The listing builds one solid part. Answer for the finished solid, in the listing's coordinates (mm). Face numbers are marked on the shaded views. Round coordinates to 2 decimals unless told otherwise and drop trailing zeros. Write each loop counter-clockwise with the first axis right and the second up, starting at its lowest first coordinate (ties: lowest second). Pieces come first, ordered by that corner, then holes.
(1) A cutting plane is placed at A-A, the plane z = 16.5. Give the vertices of the cut face in (x, y).
(2) Find the intervals of material crossed by probe 1 along Y at (x, z) = (1.5, 15.5); probe 2 along Y at (x, z) = (1.5, 18); probe 3 along X at (y, z) = (-1.25, 34.5), in increasing order.
(3) The mould has two halves that part along Y. Classify the marked faces 1 and 2: +Y half, -Y half, draft (parallel to the pull), parting line (faces both ways), or undercut.
(4) Each of these flat-tipped pins is pushed along its axis until it touches: pin 1 Ø4.5 at (x, y) = (-1.5, 1) entering from +Z; pin 2 Ø2 at (x, z) = (-1.5, 23) entering from -Y. Where does it stop, or does it pass through?
(5) A cutting plane is placed at B-B, the plane z = 24. Give the vertices of the cut face in (x, y), and give its area (3 significant figures).
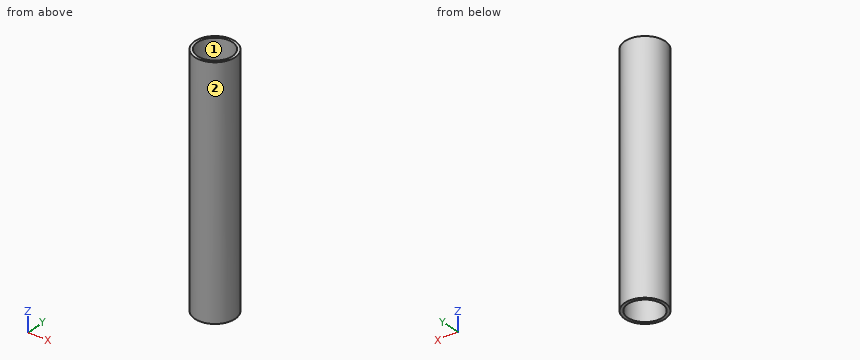
from build123d import *

# Parameters (mm, degrees)
F0_R     = 3.75
F1_DEPTH = 45
F2_R     = 3.25
F3_DEPTH = 22.5
F5_R     = 3.25
F6_DEPTH = 22.5
F7_SIZE2 = 0.49999
F7_SIZE  = 22.49999


# Not quite as in the source:
# - a fillet or chamfer that OpenCascade refuses, or shapes differently, is made with other operations: its cross-section is extruded or revolved along the edge and cut away or added
# - a fillet or chamfer is up to 0.001 mm smaller than in the source, because OpenCascade refuses the exact size


with BuildPart() as f1:
    # F0 (on Top) → F1 (new body)
    with BuildSketch(Plane.XY):
        Circle(F0_R)
    extrude(amount=F1_DEPTH)

    # F2 (on face) → F3 (cut)
    with BuildSketch(Plane.XY):
        Circle(F2_R)
    extrude(amount=F3_DEPTH, mode=Mode.SUBTRACT)

    # F4: chamfer of 25 x 0.5 on 1 edges, made by hand


with BuildPart() as f4_tool2:
    # F4_s3 → F4_t4 (revolve)
    with BuildSketch(Plane.XZ):
        Polygon((3.25, -2.5), (2.75, 22.5), (3.25, 22.5), align=None)
    revolve(axis=Axis((0, 0, 22.5), (0, 0, 1)))

    split(bisect_by=Plane.XY, keep=Keep.TOP)


with BuildPart() as f1_1:
    add(f1.part)

    # F4_t1: union F4_tool2
    add(f4_tool2.part)

    # F5 (on face) → F6 (cut)
    with BuildSketch(Plane.XY.offset(45)):
        Circle(F5_R)
    extrude(amount=-F6_DEPTH, mode=Mode.SUBTRACT)

    # F7 (size 22.5 and 0.5 in the source; OpenCascade refuses exactly that, so slightly less here)
    f7_edges = [f1_1.edges().sort_by_distance(p)[0] for p in [
        (-3.25, 0, 22.5),
    ]]
    f7_side = f1_1.faces().sort_by_distance((-3.25, 0, 33.75))[0]
    chamfer(f7_edges, length=F7_SIZE, length2=F7_SIZE2, reference=f7_side)


solid = f1_1.part
Solutions:
1. outline: circle Ø7.5 at (0, 0); hole circle Ø5.74 at (0, 0)
2. probe 1: y = -3.44 to -2.47, 2.47 to 3.44
2. probe 2: y = -3.44 to -2.41, 2.41 to 3.44
2. probe 3: x = -3.54 to -2.75, 2.75 to 3.54
3. face 1: undercut
3. face 2: parting line
4. pin 1: stops at z = 45
4. pin 2: stops at y = -3.72
5. outline: circle Ø7.5 at (0, 0); hole circle Ø5.57 at (0, 0)
5. area: 19.8 mm2
